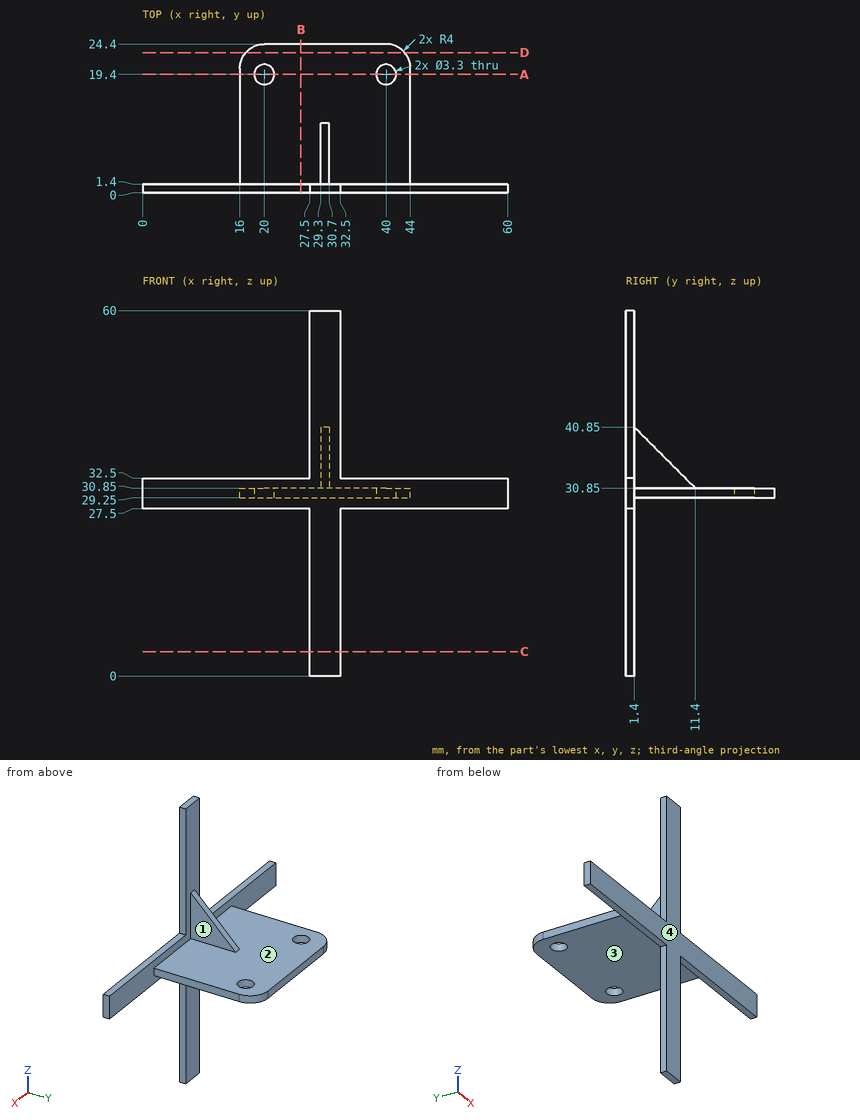
Source: three-view drawing plus pictorial views. Frame: mm from the lowest corner of the part. A direction names the side the tool comes from. Give positions to 0.01 mm unless a question says otherwise; leave off trailing zeros. Order: outer loops, then holes, each group sorted by start corner. A loop starts at its lowest first (then second) coordinate and runs counter-clockwise, first axis right, second up. Notation, with made-up numbers: M 78,22.25 L 127,22.25 A19 cw 127,50.25 Z; hole C 59,22.25 d11. An arc over 180 degrees is marked long. One line per question, with ' | ' between items. Start each with the question number.
1. Access query for the marked faces 1, 2, 3 and 4. Directions: +Z, -Z, +X, -X, +Y, -Y. A direction counts if a zero-diameter tool reaches every point of the face in a straight line with its end or side. Return the directions, or none.
2. Material intervals for probe 1 along Y at (x, z) = (40, 29.8); probe 2 along Y at (x, z) = (31, 47); probe 3 along Z at (x, y) = (40.5, 15.75), sorted ascending. Write a range as [from, to].
3. Section query B-B (x = 26). Return the cut outline in (y, z).
4. Section query D-D (y = 23). Return the cut outline in (x, z).
5. Section query C-C (z = 4). Return the cut outline in (x, y).
6. Section query A-A (y = 19.4). Return the cut outline in (x, z), and give its area (3 significant figures).
7. First-contact query: pin 1 Ø3 at (x, y) = (18, 18.5) entering from -Z; pin 2 Ø1.3 at (y, z) = (6.5, 30.5) entering from -X; pin 3 Ø1.5 at (y, z) = (1, 19) entering from +X; pin 4 Ø3 at (x, y) = (20, 19.4) entering from -Z. Flat tips, straight axial feed; report the tip coordinate or a pass-through.
Here are the results:
1) face 1: +Z, +X, +Y | face 2: +Z, +Y | face 3: -Z, +X, -X, +Y | face 4: +Z, -Z, +X, -X, -Y
2) probe 1: [0, 17.75], [21.05, 24.4] | probe 2: [0, 1.4] | probe 3: [29.25, 30.85]
3) outline: M 0,27.5 L 1.4,27.5 L 1.4,29.25 L 24.4,29.25 L 24.4,30.85 L 1.4,30.85 L 1.4,32.5 L 0,32.5 Z
4) outline: M 16.96,29.25 L 43.04,29.25 L 43.04,30.85 L 16.96,30.85 Z
5) outline: M 27.5,0 L 32.5,0 L 32.5,1.4 L 27.5,1.4 Z
6) outline: M 16,29.25 L 18.35,29.25 L 18.35,30.85 L 16,30.85 Z; M 21.65,29.25 L 38.35,29.25 L 38.35,30.85 L 21.65,30.85 Z; M 41.65,29.25 L 44,29.25 L 44,30.85 L 41.65,30.85 Z | area: 34.2 mm²
7) pin 1: z = 29.25 | pin 2: x = 16 | pin 3: x = 32.5 | pin 4: through
